Job drawing, mm, ordinate dimensions from the low corner. One solid piece. A direction names the side the tool comes from. Round coordinates to 2 decimals unless told otherwise and drop trailing zeros. Loops run counter-clockwise (first coordinate to the right, second up) from the corner with the lowest first, then second, coordinate; pieces in that order, holes last. Notation, with made-up numbers: M 52.25,73 L 81.25,73 A21 cw 81.25,88 Z; hole C -37,-28 d2. An arc over 180 degrees is marked long. Use a Markdown table: item, result. Add a question column.
(1) Flat gauge pins, fed straight in: P1, Ø1, axis at y = 19, z = 4, coming from the +X side; P2, Ø3, axis at y = 8.5, z = 15, coming from the -X side; P3, Ø1, axis at x = 9.5, z = 7, coming from the -Y side. Where does each tip first touch, or does it go through?
(2) Which spindle directions (+Z, -Z, +X, -X, +Y, -Y) get a long thin tool onto all of the face, cutting with end or side? Do the marked faces 1 and 2. Say none if no direction does.
(3) Band-saw the part on C-C, the plane z = 9. Write the cut outline in (x, y).
(4) Band-saw the part on A-A, the plane x = 12.7. Write the cut outline in (y, z) (1 decimal).
(5) Wall check: L1, parallel to Y at x = 12.7, z = 3.25; L2, parallel to Y at x = 15.5, z = 19.25 (1 decimal); L3, parallel to X at y = 10.25, z = 2. Give the ranges that are in metal, low to high.
(6) Two-plate mould, pull along X, no slides. Class the marked faces 3, 4 and 5: released by +X, released by -X, zero draft, split by the parting line, or undercut.
(7) Band-saw the part on D-D, the plane x = 20. Write the cut outline in (y, z).
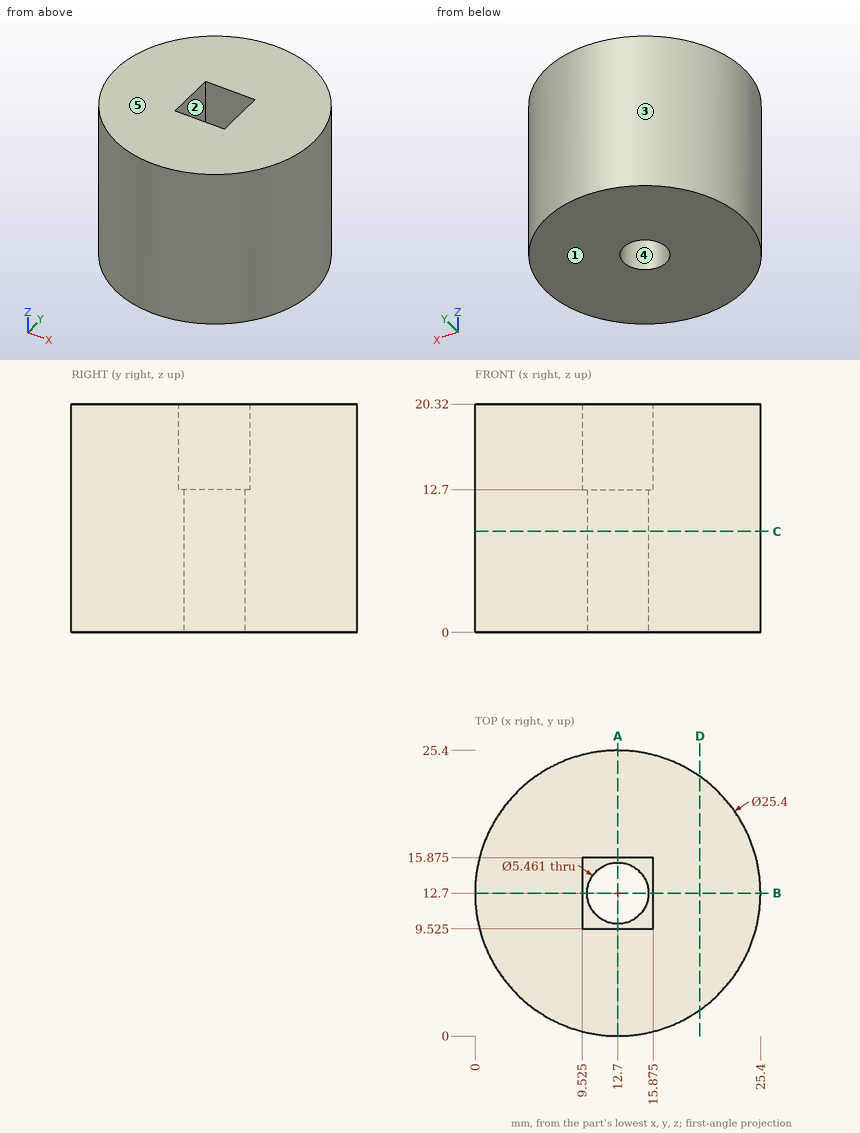
Return value:
| question | item | result |
|---|---|---|
| 1 | P1 | x = 24 |
| 1 | P2 | x = 0.29 |
| 1 | P3 | y = 0.29 |
| 2 | face 1 | -Z, +X, -X, +Y, -Y |
| 2 | face 2 | +Z |
| 3 | outline | C 12.7,12.7 d25.4; hole C 12.7,12.7 d5.46 |
| 4 | outline | M 0,0 L 10,0 L 10,12.7 L 9.5,12.7 L 9.5,20.3 L 0,20.3 Z; M 15.4,0 L 25.4,0 L 25.4,20.3 L 15.9,20.3 L 15.9,12.7 L 15.4,12.7 Z |
| 5 | L1 | 0 to 9.97, 15.43 to 25.4 |
| 5 | L2 | 0.3 to 9.5, 15.9 to 25.1 |
| 5 | L3 | 0.24 to 11.49, 13.91 to 25.16 |
| 6 | face 3 | split by the parting line |
| 6 | face 4 | undercut |
| 6 | face 5 | zero draft |
| 7 | outline | M 2.31,0 L 23.09,0 L 23.09,20.32 L 2.31,20.32 Z |
